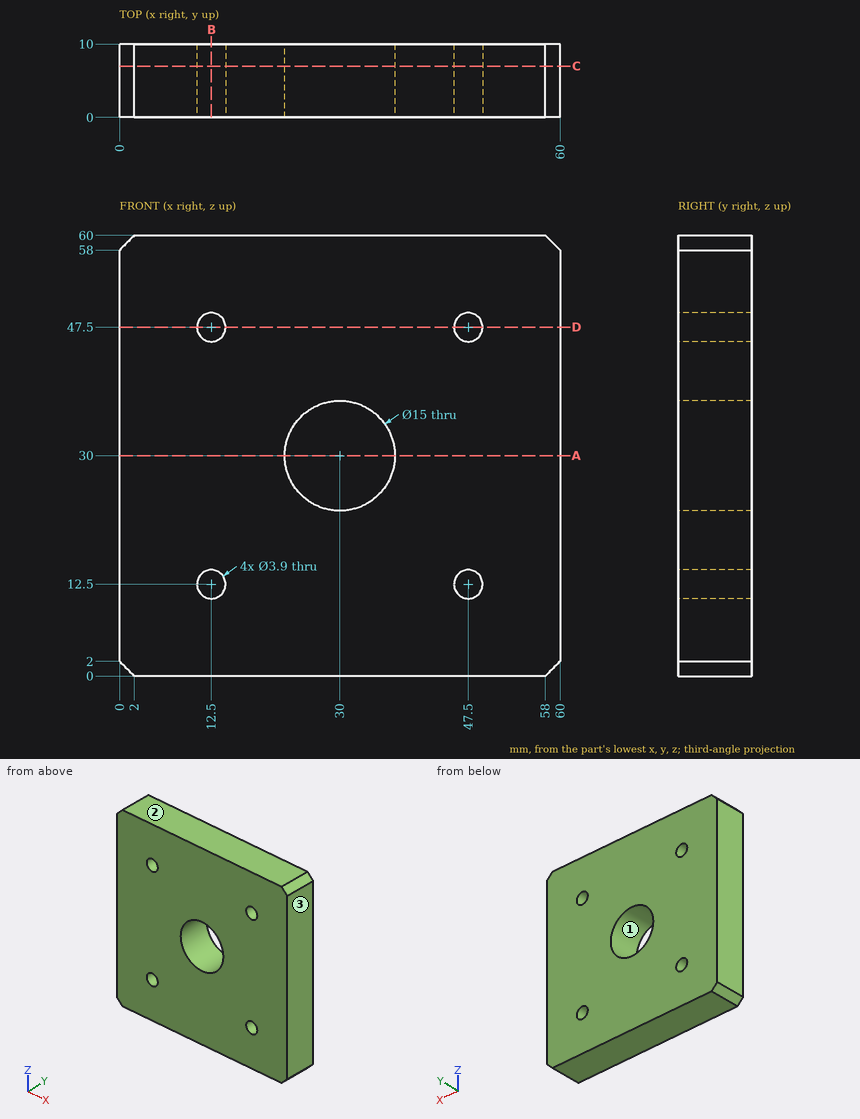
Can you work these out from the drawing? Everything is in mm from the part's minimum corner. Round coordinates to 2 decimals unless told otherwise and drop trailing zeros. Loops run counter-clockwise (first coordinate to the right, second up) from the corner with the lowest first, then second, coordinate; pieces in that order, holes last. Notation, with made-up numbers: (-21, 42.25) -> (-16, 42.25) arc R30 cw to (-16, 78.25) -> close; hole circle Ø8 at (16.5, 7.25). An arc over 180 degrees is marked (long way). Put each result on its own line as item: value.
Q1. Thinking about a two-plate mould opening in Z: for the marked faces 1, 2 and 3, which applies, pulls with the +Z half, pulls with the -Z half, needs draft (parallel to the pull), parting line crosses it, or undercut?
Checks:
face 1: undercut
face 2: pulls with the +Z half
face 3: needs draft
Q2. I want a section at C-C on y = 7. Write out the boundary of the cut face in (x, z).
Checks:
outline: (0, 2) -> (2, 0) -> (58, 0) -> (60, 2) -> (60, 58) -> (58, 60) -> (2, 60) -> (0, 58) -> close; hole circle Ø3.9 at (12.5, 12.5); hole circle Ø3.9 at (12.5, 47.5); hole circle Ø15 at (30, 30); hole circle Ø3.9 at (47.5, 12.5); hole circle Ø3.9 at (47.5, 47.5)
Q3. For pin 1 Ø2 at (x, y) = (54, 2) entering from -Z, with a flat end and sliding along its axis, tell me the tip position at first contact or that it passes through.
Checks:
pin 1: z = 0
Q4. Please list where these lines run through material, in increasing order: line 1 (Z direction, x = 12.5, y = 4); line 2 (Z direction, x = 30, y = 5.25). Write a range as from..to.
Checks:
line 1: 0..10.55, 14.45..45.55, 49.45..60
line 2: 0..22.5, 37.5..60
Q5. I want a section at A-A on z = 30. Write out the boundary of the cut face in (x, y), and give its area (3 significant figures).
Checks:
outline: (0, 0) -> (22.5, 0) -> (22.5, 10) -> (0, 10) -> close; (37.5, 0) -> (60, 0) -> (60, 10) -> (37.5, 10) -> close
area: 450 mm2
Q6. I want a section at D-D on z = 47.5. Write out the boundary of the cut face in (x, y), and give its area (3 significant figures).
Checks:
outline: (0, 0) -> (10.55, 0) -> (10.55, 10) -> (0, 10) -> close; (14.45, 0) -> (45.55, 0) -> (45.55, 10) -> (14.45, 10) -> close; (49.45, 0) -> (60, 0) -> (60, 10) -> (49.45, 10) -> close
area: 522 mm2
Q7. I want a section at B-B on x = 12.5. Write out the boundary of the cut face in (y, z).
Checks:
outline: (0, 0) -> (10, 0) -> (10, 10.55) -> (0, 10.55) -> close; (0, 14.45) -> (10, 14.45) -> (10, 45.55) -> (0, 45.55) -> close; (0, 49.45) -> (10, 49.45) -> (10, 60) -> (0, 60) -> close
